```python
from build123d import *

# Parameters (mm, degrees)
SKETCH1_W           = 31.8
SKETCH1_H           = 7.8
BOSS_EXTRUDE1_DEPTH = 4.8
SHELL2_T            = -1.6
SKETCH2_R           = 2.4
BOSS_EXTRUDE2_DEPTH = 1.8
LPATTERN1_COUNT     = 6
LPATTERN1_PITCH     = 8
SKETCH3_R           = 1.5
BOSS_EXTRUDE3_DEPTH = 8
LPATTERN2_COUNT     = 3
LPATTERN2_PITCH     = 7.95


with BuildPart() as part:
    # Sketch1 → Boss-Extrude1 (new body, symmetric)
    with BuildSketch(Plane(origin=(0, 0, 0), x_dir=(1, 0, 0), z_dir=(0, 1, 0))):
        Rectangle(SKETCH1_W, SKETCH1_H)
    extrude(amount=BOSS_EXTRUDE1_DEPTH, both=True)

    # Shell2
    shell2_openings = [part.faces().sort_by_distance(p)[0] for p in [
        (0, 0, 3.9),
    ]]
    offset(amount=SHELL2_T, openings=shell2_openings, kind=Kind.INTERSECTION)

    # Sketch2 → Boss-Extrude2 (add)
    with BuildSketch(Plane(origin=(0, 0, -3.9), x_dir=(-1, 0, 0), z_dir=(0, 0, -1))):
        with Locations((12, 0)):
            Circle(SKETCH2_R)
    boss_extrude2 = extrude(amount=BOSS_EXTRUDE2_DEPTH)

    # LPattern1: Boss-Extrude2 ×6, 2 skipped
    with Locations(*[(i * LPATTERN1_PITCH, 0, 0) for i in range(1, LPATTERN1_COUNT) if i not in (4, 5)]):
        add(boss_extrude2)

    # Sketch3 → Boss-Extrude3 (add)
    with BuildSketch(Plane.XY.offset(-2.3)):
        with Locations((-7.95, 0)):
            Circle(SKETCH3_R)
    boss_extrude3 = extrude(amount=BOSS_EXTRUDE3_DEPTH)

    # LPattern2: Boss-Extrude3 ×3
    with Locations(*[(i * LPATTERN2_PITCH, 0, 0) for i in range(1, LPATTERN2_COUNT)]):
        add(boss_extrude3)


solid = part.part
```
Design review of the part built by this model. Coordinates are the model's own, in mm. A direction names the side the tool comes from. Give positions to 0.01 mm unless a question says otherwise; leave off trailing zeros. Write each loop counter-clockwise with the first axis right and the second up, starting at its lowest first coordinate (ties: lowest second). Pieces come first, ordered by that corner, then holes.
(1) Add section A-A (z = 1.5). Give the boundary of the cut face in (x, y), and give its area (3 significant figures).
Checked values:
outline: (-15.9, -4.8) - (15.9, -4.8) - (15.9, 4.8) - (-15.9, 4.8) - close; circle Ø3 at (-7.95, 0); circle Ø3 at (0, 0); circle Ø3 at (7.95, 0); hole (-14.3, -3.2) - (14.3, -3.2) - (14.3, 3.2) - (-14.3, 3.2) - close
area: 143 mm2
(2) Tool access review of faces 5 (the face through (-9.602, 0.106, -4.787)), 6 (the face through (-6.52, 0.45, 1.64)), 7 (the face through (15.9, 0, 0)): name each direction out of +Z, -Z, +X, -X, +Y, -Y from which nothing blocks a thin tool from reaching the whole face with its end or side.
Checked values:
face 5: -Z
face 6: +Z
face 7: +Z, -Z, +X, +Y, -Y
(3) Add section D-D (y = -3.75). Give the boundary of the cut face in (x, z).
Checked values:
outline: (-15.9, -3.9) - (15.9, -3.9) - (15.9, 3.9) - (-15.9, 3.9) - close
(4) Wall thickness on line 1 along X through (y, z) = (-2, -1); line 2 along Y through (x, z) = (3, 1); line 3 along X through (y, z) = (1.5, -4): over which ranges is each line inside the solid? List them lowest first.
Checked values:
line 1: x = -15.9 to -14.3, 14.3 to 15.9
line 2: y = -4.8 to -3.2, 3.2 to 4.8
line 3: x = -13.87 to -10.13, -5.87 to -2.13, 2.13 to 5.87, 10.13 to 13.87
(5) Mouldability with a two-part tool opening along Y and no side actions: class faces 1 (the face through (0, 4.8, 0)), 2 (the face through (0, 0, -3.9)), 3 (the face through (-14.3, 0, 1)), 4 (the face through (0, 2, -2.3)) as +Y half, -Y half, draft (parallel to the pull), parting line (faces both ways), or undercut.
Checked values:
face 1: +Y half
face 2: draft
face 3: undercut
face 4: undercut
(6) Add section B-B (x = -7.95). Give the boundary of the cut face in (y, z), and give its area (3 significant figures).
Checked values:
outline: (-4.8, -3.9) - (4.8, -3.9) - (4.8, 3.9) - (3.2, 3.9) - (3.2, -2.3) - (1.5, -2.3) - (1.5, 5.7) - (-1.5, 5.7) - (-1.5, -2.3) - (-3.2, -2.3) - (-3.2, 3.9) - (-4.8, 3.9) - close
area: 59.2 mm2
(7) Add section C-C (z = 4.75). Give the boundary of the cut face in (x, y), and give its area (3 significant figures).
Checked values:
outline: circle Ø3 at (-7.95, 0); circle Ø3 at (0, 0); circle Ø3 at (7.95, 0)
area: 21.2 mm2
